Input: dimensioned drawing with shaded views. Units: mm. Origin: part minimum x, y, z. Round coordinates to 2 decimals unless told otherwise and drop trailing zeros. Order: outer loops, then holes, each group sorted by start corner. A loop starts at its lowest first (then second) coordinate and runs counter-clockwise, first axis right, second up. Notation, with made-up numbers: M 61,-32.75 L 90,-32.75 A30 ccw 90,5.25 Z; hole C -31,86 d1. An arc over 180 degrees is marked long. One line per question, with ' | ' between items.
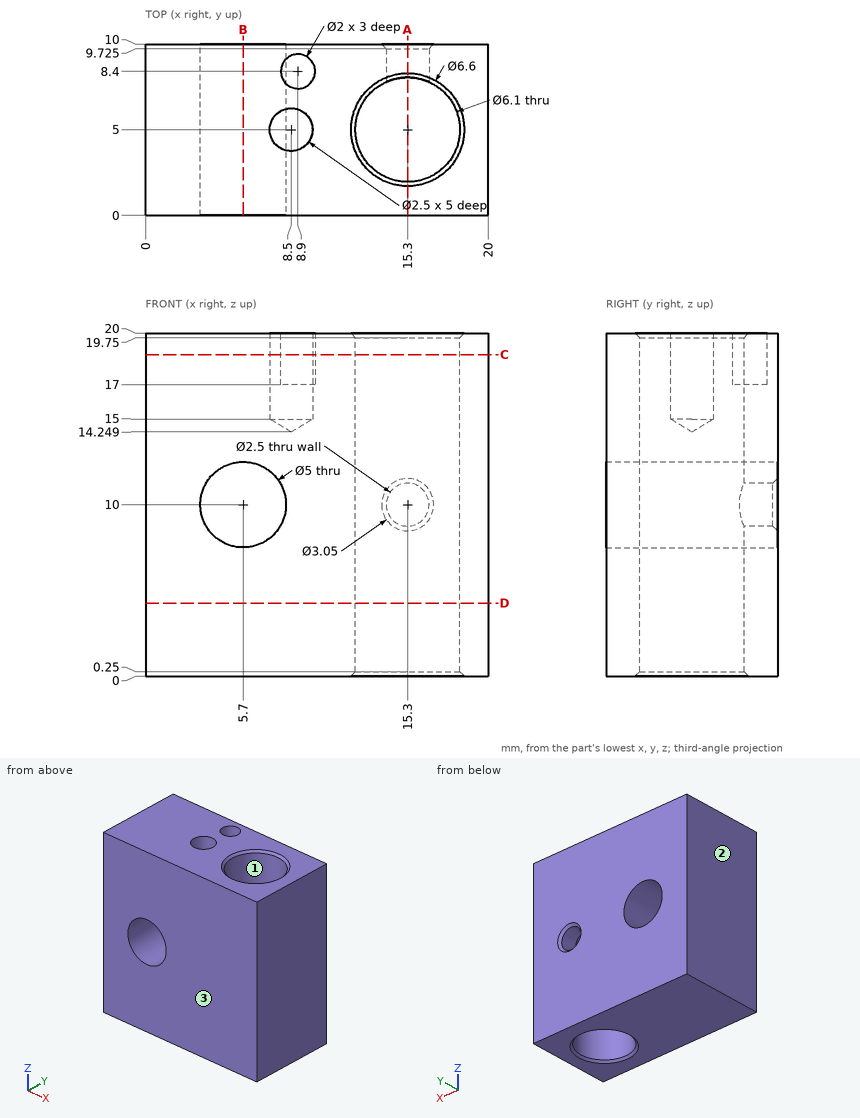
Item 1: Line query: line 1 along X through (y, z) = (5, 17.05); line 2 along X through (y, z) = (8.35, 10); line 3 along Z through (x, y) = (15.3, 8.7). Output: solid intervals per line, ascending. Write a range as from..to.
Report:
line 1: 0..7.25, 9.75..12.25, 18.35..20 | line 2: 0..3.2, 8.2..14.05, 16.55..20 | line 3: 0..8.75, 11.25..20
Item 2: Mould query, pull axis X, two halves, no side actions, for the marked faces 1, 2 and 3. Classes: +X half, -X half, draft (parallel to the pull), parting line (faces both ways), or undercut.
Report:
face 1: undercut | face 2: -X half | face 3: draft
Item 3: Section query B-B, the plane x = 5.7. Return loops of the section in (y, z), plus the area to 3 significant figures.
Report:
outline: M 0,0 L 10,0 L 10,7.5 L 0,7.5 Z; M 0,12.5 L 10,12.5 L 10,20 L 0,20 Z | area: 150 mm²
Item 4: Section query A-A, the plane x = 15.3. Return loops of the section in (y, z) (3 decimals), plus the area to 3 significant figures.
Report:
outline: M 0,0 L 1.7,0 L 1.95,0.25 L 1.95,19.75 L 1.7,20 L 0,20 Z; M 8.05,0.25 L 8.3,0 L 10,0 L 10,8.475 L 9.725,8.75 L 8.05,8.75 Z; M 8.05,11.25 L 9.725,11.25 L 10,11.525 L 10,20 L 8.3,20 L 8.05,19.75 Z | area: 72.9 mm²
Item 5: Section query C-C, the plane z = 18.75. Return loops of the section in (x, y), plus the area to 3 significant figures.
Report:
outline: M 0,0 L 20,0 L 20,10 L 0,10 Z; hole C 8.5,5 d2.5; hole C 8.9,8.4 d2; hole C 15.3,5 d6.1 | area: 163 mm²
Item 6: First-contact query: pin 1 (1.5 mm diameter, centred on x = 15.3, z = 10, fed in from +Y). Flat tip, straight axial feed; report the tip coordinate or a pass-through.
Report:
pin 1: y = 2.04
Item 7: Section query D-D, the plane z = 4.25. Return loops of the section in (x, y), plus the area to 3 significant figures.
Report:
outline: M 0,0 L 20,0 L 20,10 L 0,10 Z; hole C 15.3,5 d6.1 | area: 171 mm²
